Print and shaded views of the part. All mm, measured from the part's lowest x, y and z. Round coordinates to 2 decimals unless told otherwise and drop trailing zeros. Loops run counter-clockwise (first coordinate to the right, second up) from the corner with the lowest first, then second, coordinate; pieces in that order, holes last. Notation, with made-up numbers: (38.5, 37.5) -> (67.5, 37.5) arc R15 ccw to (67.5, 42.5) -> close; hole circle Ø5 at (74, 57). An arc over 180 degrees is marked (long way). Use a Markdown table: item, result.
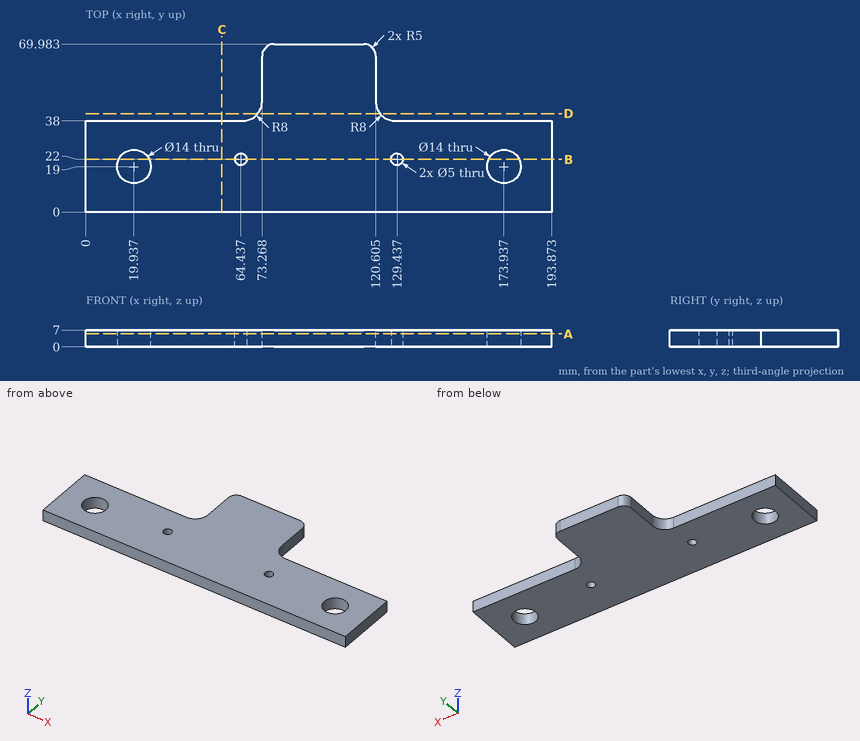
Q1. Band-saw the part on A-A, the plane z = 5.5. Give the cut face in (x, y) (1 decimal), plus the area to 3 significant figures.
Results list:
| item | result |
|---|---|
| outline | (0, 0) -> (193.9, 0) -> (193.9, 38) -> (128.6, 38) arc R8 cw to (120.6, 46) -> (120.6, 65) arc R5 ccw to (115.6, 70) -> (78.3, 70) arc R5 ccw to (73.3, 65) -> (73.3, 46) arc R8 cw to (65.3, 38) -> (0, 38) -> close; hole circle Ø14 at (19.9, 19); hole circle Ø5 at (64.4, 22); hole circle Ø5 at (129.4, 22); hole circle Ø14 at (173.9, 19) |
| area | 8,550 mm² |
Q2. Band-saw the part on C-C, the plane x = 56.5. Give the cut face in (y, z), plus the area to 3 significant figures.
Results list:
| item | result |
|---|---|
| outline | (0, 0) -> (38, 0) -> (38, 7) -> (0, 7) -> close |
| area | 266 mm² |
Q3. Band-saw the part on B-B, the plane y = 22. Give the cut face in (x, z).
Results list:
| item | result |
|---|---|
| outline | (0, 0) -> (13.61, 0) -> (13.61, 7) -> (0, 7) -> close; (26.26, 0) -> (61.94, 0) -> (61.94, 7) -> (26.26, 7) -> close; (66.94, 0) -> (126.94, 0) -> (126.94, 7) -> (66.94, 7) -> close; (131.94, 0) -> (167.61, 0) -> (167.61, 7) -> (131.94, 7) -> close; (180.26, 0) -> (193.87, 0) -> (193.87, 7) -> (180.26, 7) -> close |
Q4. Flat gauge pins, fed straight in: pin 1 (8.5 mm diameter, centred on x = 19.94, y = 19, fed in from -Z); pin 2 (4 mm diameter, centred on y = 46.5, z = 4, fed in from -X); pin 3 (3.5 mm diameter, centred on x = 175.5, z = 2.5, fed in from +Y). Where does each tip first touch, or does it go through?
Results list:
| item | result |
|---|---|
| pin 1 | passes through |
| pin 2 | stops at x = 73.13 |
| pin 3 | stops at y = 38 |
Q5. Band-saw the part on D-D, the plane y = 41. Give the cut face in (x, z), plus the area to 3 significant figures.
Results list:
| item | result |
|---|---|
| outline | (71.51, 0) -> (122.36, 0) -> (122.36, 7) -> (71.51, 7) -> close |
| area | 356 mm² |
Q6. Drill centre lines: L1, parallel to Y at x = 163.5, z = 3; L2, parallel to X at y = 46, z = 5.5 (1 decimal); L3, parallel to X at y = 21, z = 4.5 (1 decimal). Where is each one in solid material? Low to high. Write a range as from..to.
Results list:
| item | result |
|---|---|
| L1 | y = 0..38 |
| L2 | x = 73.3..120.6 |
| L3 | x = 0..13.2, 26.6..62.1, 66.7..127.1, 131.7..167.2, 180.6..193.9 |
